The listing builds one solid part. Answer for the finished solid, in the listing's coordinates (mm). Face numbers are marked on the shaded views. A direction names the side the tool comes from. Give positions to 0.01 mm unless a question says otherwise; leave off trailing zeros. Loops run counter-clockwise (first coordinate to the right, second up) from the corner with the lowest first, then second, coordinate; pieces in that order, holes last. Notation, with made-up numbers: M 38.5,87.25 L 60.5,87.25 A23 ccw 60.5,103.25 Z; hole C 23.25,83 d1. An arc over 180 degrees is marked long. One line per item, written item: value. Start each with the question number.
Q1. A cutting plane is placed at A-A, the plane z = -292.5. Determine the outline of the cut face in (x, y).
Q2. Consider L1, parallel to X at y = 62, z = 89; L2, parallel to Z at x = 7.5, y = 64.5; L3, parallel to X at y = 7, z = -121.5. Determine where each line is inside the solid, lowest interval first.
Q3. For the marked faces 3 and 4, determine the directions among +Z, -Z, +X, -X, +Y, -Y from which every point of the face is accessible in a straight line to the end or side of a thin tool.
Q4. A cutting plane is placed at D-D, the plane y = 15. Determine the outline of the cut face in (x, z), and give its area (3 significant figures).
Q5. A cutting plane is placed at B-B, the plane y = 90. Determine the outline of the cut face in (x, z).
Q6. The mould has two halves that part along X. Classify the marked faces 1 and 2: +X half, -X half, draft (parallel to the pull), parting line (faces both ways), or undercut.
Q7. A cutting plane is placed at C-C, the plane x = 269.5. Determine the outline of the cut face in (y, z).
from build123d import *

# Parameters (mm, degrees)
SKETCH1_W           = 889
SKETCH1_H           = 889
SKETCH1_W_2         = 711.2
SKETCH1_H_2         = 711.2
BOSS_EXTRUDE1_DEPTH = 139.7
FILLET2_R           = 25.4


with BuildPart() as part:
    # Sketch1 → Boss-Extrude1 (new body)
    with BuildSketch(Plane(origin=(0, 0, 0), x_dir=(1, 0, 0), z_dir=(0, 1, 0))):
        with Locations((-38.710886076, -21.155949367)):
            Rectangle(SKETCH1_W, SKETCH1_H)
        with Locations((-38.710886076, -21.155949367)):
            Rectangle(SKETCH1_W_2, SKETCH1_H_2, mode=Mode.SUBTRACT)
    extrude(amount=BOSS_EXTRUDE1_DEPTH)

    # Fillet2
    fillet2_edges = [part.edges().sort_by_distance(p)[0] for p in [
        (-483.210886076, 139.7, 21.155949367),
        (-38.710886076, 139.7, 465.655949367),
        (405.789113924, 139.7, 21.155949367),
        (-38.710886076, 0, 465.655949367),
        (-483.210886076, 0, 21.155949367),
        (-38.710886076, 0, -423.344050633),
        (405.789113924, 0, 21.155949367),
        (405.789113924, 69.85, 465.655949367),
        (-483.210886076, 69.85, 465.655949367),
        (-483.210886076, 69.85, -423.344050633),
        (405.789113924, 69.85, -423.344050633),
        (-38.710886076, 139.7, -423.344050633),
    ]]
    fillet(fillet2_edges, radius=FILLET2_R)


solid = part.part
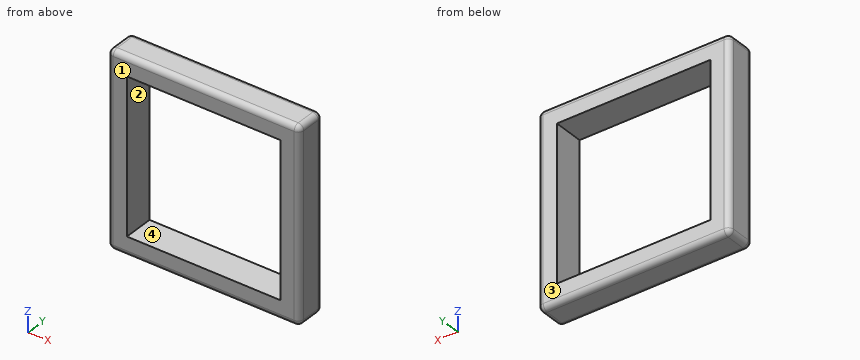
Answer block:
1. outline: M -483.21,25.4 A25.4 ccw -457.81,0 L -394.31,0 L -394.31,139.7 L -457.81,139.7 A25.4 ccw -483.21,114.3 Z; M 316.89,0 L 380.39,0 A25.4 ccw 405.79,25.4 L 405.79,114.3 A25.4 ccw 380.39,139.7 L 316.89,139.7 Z
2. L1: -483.21 to -394.31, 316.89 to 405.79
2. L2: -423.34 to -334.44, 376.76 to 465.66
2. L3: -475.32 to -394.31, 316.89 to 397.9
3. face 3: +Z, -Z, +X, -X, +Y
3. face 4: +Y, -Y
4. outline: M -480.98,-397.94 A23.17 ccw -457.81,-421.12 L 380.39,-421.12 A23.17 ccw 403.56,-397.94 L 403.56,440.26 A23.17 ccw 380.39,463.43 L -457.81,463.43 A23.17 ccw -480.98,440.26 Z; hole M -394.31,-334.44 L 316.89,-334.44 L 316.89,376.76 L -394.31,376.76 Z
4. area: 276,000 mm^2
5. outline: M -483.21,-397.94 A25.4 ccw -457.81,-423.34 L 380.39,-423.34 A25.4 ccw 405.79,-397.94 L 405.79,440.26 A25.4 ccw 380.39,465.66 L -457.81,465.66 A25.4 ccw -483.21,440.26 Z; hole M -394.31,-334.44 L 316.89,-334.44 L 316.89,376.76 L -394.31,376.76 Z
6. face 1: draft
6. face 2: undercut
7. outline: M 0,-397.94 A25.4 ccw 25.4,-423.34 L 114.3,-423.34 A25.4 ccw 139.7,-397.94 L 139.7,-334.44 L 0,-334.44 Z; M 0,376.76 L 139.7,376.76 L 139.7,440.26 A25.4 ccw 114.3,465.66 L 25.4,465.66 A25.4 ccw 0,440.26 Z
